Here's how the part is built. I have some questions about the finished solid (model axes, mm). Coordinates: 2 decimals unless noted, no trailing zeros. Order: outer loops, then holes, each group sorted by start corner. A loop starts at its lowest first (then second) coordinate and runs counter-clockwise, first axis right, second up. Notation, with made-up numbers: (49.5, -28.75) - (96.5, -28.75) arc R13 cw to (96.5, -4.75) - close; hole circle Ø7 at (1.25, 1). An arc over 180 degrees is marked (long way). Answer as CSV lines item,"result". Start each with the question number.
Q1. I need wall thicknesses on line 1 (X direction, y = -0.6, z = -19.5); line 2 (X direction, y = -0.6, z = -42); line 3 (Z direction, x = -12, y = -0.85). Which ranges of each line are inside material? Lowest first, please.
Q2. Suppose I cut it at B-B (x = 11.5). Please give me the cut outline in (y, z).
Q3. For pin 1 Ø8 at (x, z) = (-7, -47.5) entering from +Y, with a flat end and sliding along its axis, tell me the tip position at first contact or that it passes through.
Q4. Suppose I cut it at A-A (z = 0). Please give me the cut outline in (x, y).
Q5. Suppose I cut it at C-C (x = 3.5). Please give me the cut outline in (y, z), then the cut area to 3 significant figures.
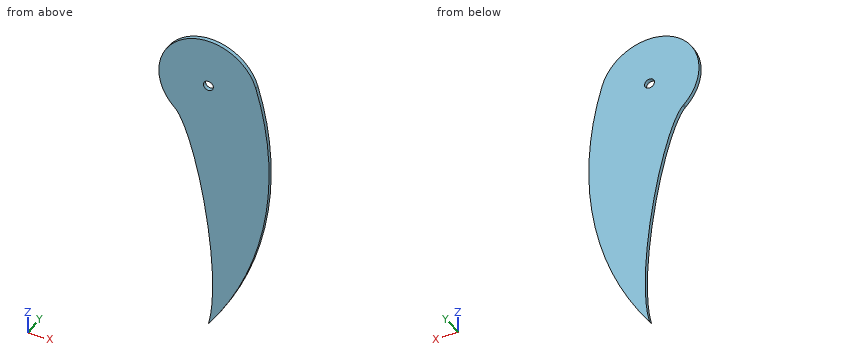
from build123d import *

# Parameters (mm, degrees)
F0_R     = 1.5
F1_DEPTH = 1.2


# Not quite as in the source:
# - a feature names something its author has since deleted; it is built from what else it names


with BuildPart() as f1:
    # F0 (on Front) → F1 (new body)
    with BuildSketch(Plane.XZ):
        with BuildLine():
            ThreePointArc((-10.1224102731, -11.0696346038), (6.0482991784, -13.7265464356), (15, 0))
            ThreePointArc((15, 0), (14.8438679143, 2.1586072693), (14.3787219542, 4.2722774913))
            ThreePointArc((14.3787219542, 4.2722774913), (-7.8146967903, 12.8035352179), (-10.3730753026, -10.8350961587))
            add(Edge.make_bspline(
                [(-10.1224102731, -11.0696346038), (-10.2063109594, -10.9847137567), (-10.2898772286, -10.9064839504), (-10.3730753026, -10.8350961587)],
                knots=[69.0284339282, 69.0284339282, 69.0284339282, 69.0284339282, 69.9384344593, 69.9384344593, 69.9384344593, 69.9384344593], degree=3))
        make_face()
        Circle(F0_R, mode=Mode.SUBTRACT)
        with BuildLine():
            ThreePointArc((14.3787219542, 4.2722774913), (14.8438679143, 2.1586072693), (15, 0))
            ThreePointArc((15, 0), (6.0482991784, -13.7265464356), (-10.1224102731, -11.0696346038))
            add(Edge.make_bspline(
                [(0, -80), (4.5304750858, -62.4535454421), (-3.758092031, -17.5113375297), (-10.1224102731, -11.0696346038)],
                knots=[0, 0, 0, 0, 69.0284339282, 69.0284339282, 69.0284339282, 69.0284339282], degree=3))
            ThreePointArc((0, -80), (17.0066443872, -39.5389078142), (14.3787219542, 4.2722774913))
        make_face()
    extrude(amount=F1_DEPTH)


solid = f1.part
Here are the results:
1,line 1,"x = -6.03 to 18.31"
1,line 2,"x = -0.87 to 16.55"
1,line 3,"z = -9 to 9"
2,outline,"(-1.2, -59.11) - (0, -59.11) - (0, 9.63) - (-1.2, 9.63) - close"
3,pin 1,"passes through"
4,outline,"(-15, -1.2) - (-1.5, -1.2) - (-1.5, 0) - (-15, 0) - close; (1.5, -1.2) - (15.54, -1.2) - (15.54, 0) - (1.5, 0) - close"
5,outline,"(-1.2, -74.82) - (0, -74.82) - (0, 14.59) - (-1.2, 14.59) - close"
5,area,"107 mm²"
